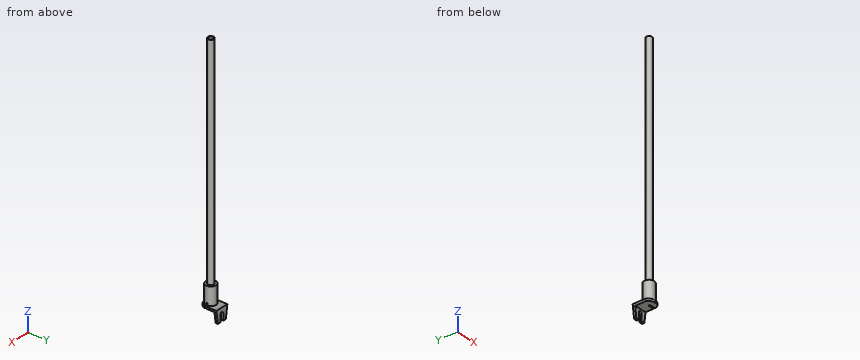
```python
from build123d import *

# Parameters (mm, degrees)
ESQUISSE1_R             = 3.5
ESQUISSE1_R_2           = 1
BASE_EXTRUSION_DEPTH    = 12
ESQUISSE2_R             = 2
ESQUISSE2_R_2           = 1.5
BOSS_EXTRU_1_DEPTH      = 150
BOSS_EXTRU_2_DEPTH      = 4.5
CONG_1_R                = 4
ESQUISSE4_W             = 7
ESQUISSE4_H             = 1
ENL_V_MAT_EXTRU_1_DEPTH = 3
ENL_V_MAT_EXTRU_2_DEPTH = 12.5


with BuildPart() as part:
    # Esquisse1 → Base-Extrusion (new body)
    with BuildSketch(Plane.XY):
        Circle(ESQUISSE1_R)
        Circle(ESQUISSE1_R_2, mode=Mode.SUBTRACT)
    extrude(amount=BASE_EXTRUSION_DEPTH)

    # Esquisse2 → Boss.-Extru.1 (add)
    with BuildSketch(Plane.XY.offset(12)):
        Circle(ESQUISSE2_R)
        Circle(ESQUISSE2_R_2, mode=Mode.SUBTRACT)
    extrude(amount=BOSS_EXTRU_1_DEPTH)

    # Esquisse3 → Boss.-Extru.2 (add, symmetric)
    with BuildSketch(Plane(origin=(0, 0, 0), x_dir=(0, 0, -1), z_dir=(1, 0, 0))):
        Polygon((0, 0), (0, 7.5), (11.5, 7.5), (11.5, 6), (1.5, 6), (1.5, -4), (0, -4), align=None)
    extrude(amount=BOSS_EXTRU_2_DEPTH, both=True)

    # Congé1
    cong_1_edges = [part.edges().sort_by_distance(p)[0] for p in [
        (4.5, -4, -0.75),
        (-4.5, -4, -0.75),
    ]]
    fillet(cong_1_edges, radius=CONG_1_R)

    # Esquisse4 → Enlèv. mat.-Extru.1 (cut)
    with BuildSketch(Plane(origin=(0, 0, -1.5), x_dir=(-1, 0, 0), z_dir=(0, 0, -1))):
        with Locations((-3.5, 0)):
            Rectangle(ESQUISSE4_W, ESQUISSE4_H)
    extrude(amount=-ENL_V_MAT_EXTRU_1_DEPTH, mode=Mode.SUBTRACT)

    # Esquisse5 → Enlèv. mat.-Extru.2 (cut, through all)
    with BuildSketch(Plane(origin=(0, 7.5, 0), x_dir=(-1, 0, 0), z_dir=(0, 1, 0))):
        with BuildLine():
            Line((1.155842945, -8.594721571), (1.155842945, -3.98824613))
            ThreePointArc((1.155842945, -3.98824613), (0, -2.832403184), (-1.155842945, -3.98824613))
            Line((-1.155842945, -3.98824613), (-1.155842945, -8.594721571))
            Line((-1.155842945, -8.594721571), (-3.272534799, -8.594721571))
            Line((-3.272534799, -8.594721571), (-4.5, 0))
            Line((-4.5, 0), (-6, 0))
            Line((-6, 0), (-6, -13))
            Line((-6, -13), (6, -13))
            Line((6, -13), (6, 0))
            Line((6, 0), (4.5, 0))
            Line((4.5, 0), (3.272534799, -8.594721571))
            Line((3.272534799, -8.594721571), (1.155842945, -8.594721571))
        make_face()
    extrude(amount=-ENL_V_MAT_EXTRU_2_DEPTH, mode=Mode.SUBTRACT)


solid = part.part
```
Verification items for the finished model (mm, model axes). Round coordinates to 2 decimals unless told otherwise and drop trailing zeros. Write each loop counter-clockwise with the first axis right and the second up, starting at its lowest first coordinate (ties: lowest second). Pieces come first, ordered by that corner, then holes.
1. Section check B-B on z = 124. Enter the section's corners in (x, y), plus the area to 3 significant figures.
2. Gauge pin test, flat ends, axial feed: P1, Ø0.5, axis at y = 0, z = -0.5, coming from the +X side; P2, Ø4.5, axis at x = -1.5, y = 3, coming from the +Z side; P3, Ø3, axis at y = 4.5, z = 16.5, coming from the -X side; P4, Ø1, axis at x = 0, y = 0.5, coming from the -Z side. Record the tip position at first contact, or that the pin passes through.
3. Section check A-A on z = 5. Enter the section's corners in (x, y), plus the area to 3 significant figures.
4. Scan lines: L1, parallel to Y at x = 0, z = 112; L2, parallel to Y at x = 0, z = 3.75; L3, parallel to Z at x = 0.25, y = 1.25. Record each from-to range of solid material in increasing order.
Answer:
1. outline: circle Ø4 at (0, 0); hole circle Ø3 at (0, 0)
1. area: 5.50 mm2
2. P1: stops at x = 0
2. P2: stops at z = 162
2. P3: passes through
2. P4: stops at z = -1.5
3. outline: circle Ø7 at (0, 0); hole circle Ø2 at (0, 0)
3. area: 35.3 mm2
4. L1: y = -2 to -1.5, 1.5 to 2
4. L2: y = -3.5 to -1, 1 to 3.5
4. L3: z = -1.5 to 12
